```python
from build123d import *

# Parameters (mm, degrees)
SKETCH1_R           = 2.023987864
SKETCH1_R_2         = 2.023043511
BOSS_EXTRUDE1_DEPTH = 6


with BuildPart() as part:
    # Sketch1 → Boss-Extrude1 (new body)
    with BuildSketch(Plane.XY):
        with BuildLine():
            ThreePointArc((40.235925581, 13.621604134), (57.203735223, 20.491828906), (72.938383073, 29.847437358))
            Line((72.938383073, 29.847437358), (74.156447949, 30.67709719))
            ThreePointArc((74.156447949, 30.67709719), (84.681220688, 26.906078771), (78.020019153, 17.927224989))
            Line((78.020019153, 17.927224989), (13.323500668, -3.100956986))
            ThreePointArc((13.323500668, -3.100956986), (6.814395622, -5.556227345), (0, -6.956517793))
            ThreePointArc((0, -6.956517793), (-6.956517793, 0), (0, 6.956517793))
            ThreePointArc((0, 6.956517793), (20.269294729, 9.375497313), (40.235925581, 13.621604134))
        make_face()
        with Locations((78.020019153, 24.887546661)):
            Circle(SKETCH1_R, mode=Mode.SUBTRACT)
        Circle(SKETCH1_R_2, mode=Mode.SUBTRACT)
    extrude(amount=BOSS_EXTRUDE1_DEPTH)


solid = part.part
```
Design review of the part built by this model. Coordinates are the model's own, in mm. Coordinates: 2 decimals unless noted, no trailing zeros. Order: outer loops, then holes, each group sorted by start corner. A loop starts at its lowest first (then second) coordinate and runs counter-clockwise, first axis right, second up.
1) Mouldability with a two-part tool opening along X and no side actions: class faces 1 (the cylindrical face through (19.99, 9.33, 2.96)), 2 (the cylindrical face through (6.91, -5.53, 2.96)), 3 (the flat face through (39, 13, 0)), 4 (the cylindrical face through (76.41, 23.66, 2.96)) as +X half, -X half, draft (parallel to the pull), parting line (faces both ways), or undercut.
2) Take a section at A-A, the plane y = 0. Give the boundary of the cut face in (x, z), and give its area (3 significant figures).
3) Clearance check with flat-ended pins moving along their axes: pin 1 (3.5 mm diameter, centred on x = 78.02, y = 24.89, fed in from -Z); pin 2 (1.5 mm diameter, centred on y = 26.5, z = 2, fed in from -X); pin 3 (1 mm diameter, centred on x = 52.5, z = 3, fed in from +Y). State where each tip first meets the part, or that it passes through.
4) Take a section at C-C, the plane x = 20. Give the boundary of the cut face in (y, z), and give its area (3 significant figures).
5) Take a section at B-B, the plane z = 2.4. Give the boundary of the cut face in (x, y).
6) Take a section at D-D, the plane y = 16.5. Give the boundary of the cut face in (x, z).
7) Wall thickness on line 1 along Y through (x, z) = (5, 1.05); line 2 along Y through (x, z) = (3.5, 2.3); line 3 along X through (y, z) = (30, 2.3): over which ranges is each line inside the solid? List them lowest first.
Returned:
1. face 1: -X half
1. face 2: +X half
1. face 3: draft
1. face 4: undercut
2. outline: (-6.96, 0) - (-2.02, 0) - (-2.02, 6) - (-6.96, 6) - close; (2.02, 0) - (22.86, 0) - (22.86, 6) - (2.02, 6) - close
2. area: 155 mm2
3. pin 1: passes through
3. pin 2: stops at x = 66.7
3. pin 3: stops at y = 18.51
4. outline: (-0.93, 0) - (9.33, 0) - (9.33, 6) - (-0.93, 6) - close
4. area: 61.6 mm2
5. outline: (0, -6.96) arc R44.07 ccw to (13.32, -3.1) - (78.02, 17.93) arc R6.96 ccw (long way) to (74.16, 30.68) - (72.94, 29.85) arc R120.78 cw to (40.24, 13.62) arc R224.99 cw to (0, 6.96) arc R6.96 ccw to start; hole circle Ø4.05 at (0, 0); hole circle Ø4.05 at (78.02, 24.89)
6. outline: (48.27, 0) - (73.63, 0) - (73.63, 6) - (48.27, 6) - close
7. line 1: y = -6.04 to 7.38
7. line 2: y = -6.38 to 7.24
7. line 3: x = 73.16 to 82.74
